Source: three-view drawing plus pictorial views. Frame: mm from the lowest corner of the part. Coordinates: 2 decimals unless noted, no trailing zeros. Loops run counter-clockwise (first coordinate to the right, second up) from the corner with the lowest first, then second, coordinate; pieces in that order, holes last. Notation, with made-up numbers: (-14, -25) - (27, -25) arc R9 cw to (27, -10) - close; hole circle Ø7 at (40.5, 80). An arc over 180 degrees is marked (long way). Return JSON: item names as keys, results as strings.
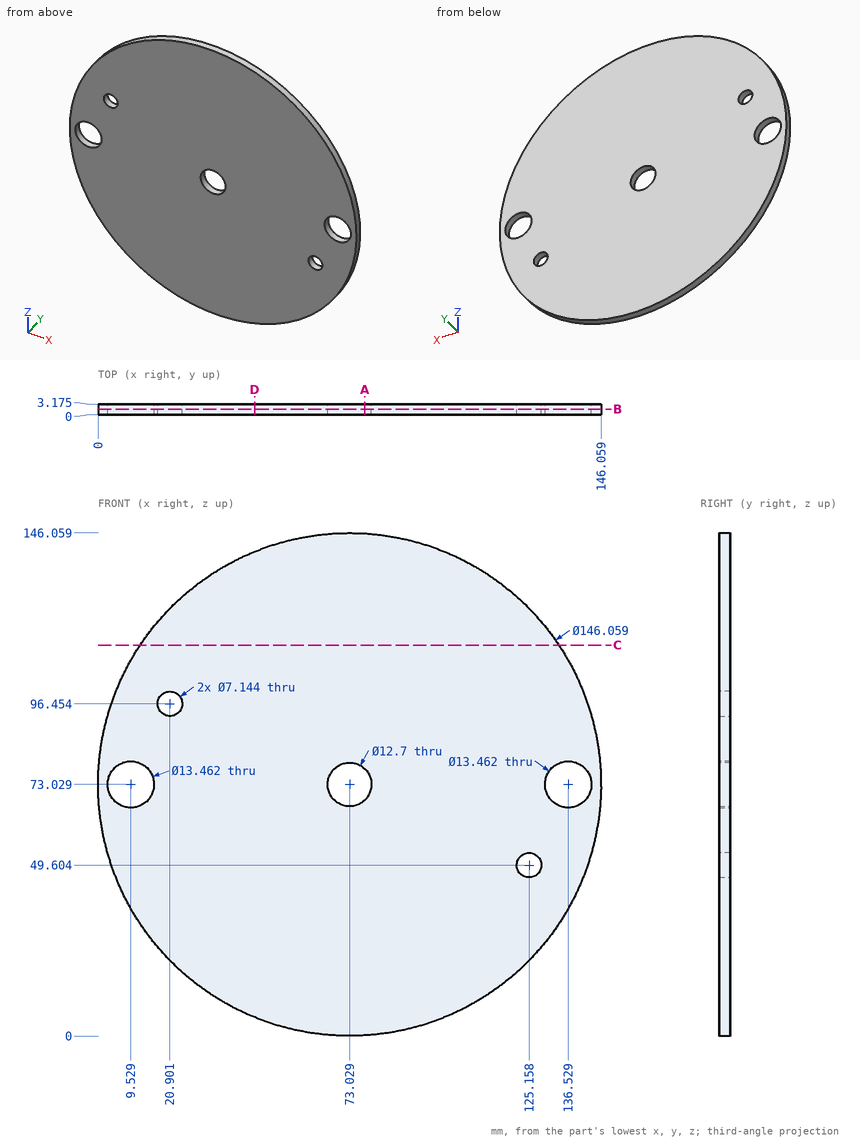
Item 1: Section query A-A, the plane x = 77.5. Return loops of the section in (y, z) (1 decimal), and give its area (3 significant figures).
Worked out:
{"outline": "(0, 0.1) - (3.2, 0.1) - (3.2, 68.5) - (0, 68.5) - close; (0, 77.5) - (3.2, 77.5) - (3.2, 145.9) - (0, 145.9) - close", "area": "434 mm^2"}
Item 2: Section query D-D, the plane x = 45.5. Return loops of the section in (y, z) (1 decimal).
Worked out:
{"outline": "(0, 5.4) - (3.2, 5.4) - (3.2, 140.7) - (0, 140.7) - close"}
Item 3: Section query B-B, the plane y = 1.7. Count the separate pieces of the cut face and the enclosed holes in it, and give its area (3 significant figures).
Worked out:
{"separate pieces": "1", "enclosed holes": "5", "area": "16,300 mm^2"}
Item 4: Ray query, probe 1 along X at (y, z) = (0.4, 74) (1 decimal); probe 2 along X at (y, z) = (2.7, 77.5) (1 decimal); probe 3 along Z at (x, y) = (71, 2.55) (1 decimal). Return the intervals inside material, ascending. Write a range as from..to.
Worked out:
{"probe 1": "0..2.9, 16.2..66.8, 79.3..129.9, 143.2..146.1", "probe 2": "0.1..4.5, 14.6..68.5, 77.5..131.5, 141.6..145.9", "probe 3": "0..67, 79..146"}
Item 5: First-contact query: pin 1 Ø4.5 at (x, z) = (20.9, 96.45) entering from +Y; pin 2 Ø1.5 at (x, y) = (20.5, 2.5) entering from +Z; pin 3 Ø1 at (x, y) = (16, 0.5) entering from -Z (1 decimal); pin 4 Ø1 at (y, z) = (1, 126) entering from -X (1 decimal). Flat tips, straight axial feed; report the tip coordinate or a pass-through.
Worked out:
{"pin 1": "through", "pin 2": "z = 124.53", "pin 3": "z = 26.8", "pin 4": "x = 22.2"}
Item 6: Section query C-C, the plane z = 113.5. Return loops of the section in (x, y) (1 decimal), and give its area (3 significant figures).
Worked out:
{"outline": "(12.2, 0) - (133.8, 0) - (133.8, 3.2) - (12.2, 3.2) - close", "area": "386 mm^2"}
